The listing builds one solid part. Answer for the finished solid, in the listing's coordinates (mm). A direction names the side the tool comes from. Coordinates: 2 decimals unless noted, no trailing zeros. Write each loop counter-clockwise with the first axis right and the second up, starting at its lowest first coordinate (ties: lowest second). Pieces come first, ordered by that corner, then holes.
(1) For a pull along Y with two mould halves and no side action, classify faces 4 (the cylindrical face through (15.376, 0.066, 6.365)), 5 (the cylindrical face through (12.5, 2.24, -0.05)), 6 (the cylindrical face through (-19.974, -0.068, -6.365)), 7 (the cylindrical face through (6.365, 0.066, -15.376)) as +Y half, -Y half, draft (parallel to the pull), parting line (faces both ways), or undercut.
(2) The part is cut by section A-A on z = 0. Determine the outline of the cut face in (x, y), plus the area to 3 significant figures.
(3) The part is cut by section C-C on z = 5.5. Determine the outline of the cut face in (x, y) (3 decimals), plus the area to 3 significant figures.
(4) The part is cut by section D-D on y = -1. Give the number of separate pieces and of enclosed holes in the cut face, plus the area to 3 significant figures.
(5) The part is cut by section B-B on x = 16. Determine the outline of the cut face in (y, z).
(6) Which of the six approach directions +Z, -Z, +X, -X, +Y, -Y give full straight-line access (tool end or side, diameter ignored) to faces 1 (the cylindrical face through (12.5, -2.24, -0.05)), 2 (the cylindrical face through (-12.5, -2.24, 0.05)), 3 (the cylindrical face through (0.05, 2.24, 12.5))?
(7) Straight lines are drawn through the part: line 1 (X direction, y = 0, z = 7.45) (3 decimals); line 2 (X direction, y = 2.75, z = 15.5). For each, find the intervals that lie inside material, in ascending order.
(8) Given P1, Ø10, axis at x = -16, z = -14.5, coming from the -Y side; P2, Ø1.9, axis at x = -17.5, y = -1, coming from the -Z side; P3, Ø2, axis at y = -1.5, z = 12.5, coming from the -X side; P4, Ø1, axis at y = -2, z = -7.5, coming from the -X side, each flat-ended and moving along its own axis, determine where each tip first touches the part or whether it passes through.
from build123d import *

# Parameters (mm, degrees)
SKETCH1_R           = 2.5
BOSS_EXTRUDE1_DEPTH = 3.1
CUT_EXTRUDE1_START  = -30.25
SKETCH2_R           = 1.5
CUT_EXTRUDE1_DEPTH  = 42.7
CIRPATTERN1_COUNT   = 4
FILLET1_R           = 3
CHAMFER1_SIZE       = 1
CHAMFER3_SIZE       = 0.5


with BuildPart() as part:
    # Sketch1 → Boss-Extrude1 (new body, symmetric)
    with BuildSketch(Plane(origin=(0, 0, 0), x_dir=(1, 0, 0), z_dir=(0, 1, 0))):
        Polygon((-8.9, -13.4), (-8.9, -20.35), (-3.9, -20.35), (-3.9, -13.4), (3.9, -13.4), (3.9, -20.35), (8.9, -20.35), (8.9, -13.4), (13.4, -8.9), (20.35, -8.9), (20.35, -3.9), (13.4, -3.9), (13.4, 3.9), (20.35, 3.9), (20.35, 8.9), (13.4, 8.9), (8.9, 13.4), (8.9, 20.35), (3.9, 20.35), (3.9, 13.4), (-3.9, 13.4), (-3.9, 20.35), (-8.9, 20.35), (-8.9, 13.4), (-13.4, 8.9), (-20.35, 8.9), (-20.35, 3.9), (-13.4, 3.9), (-13.4, -3.9), (-20.35, -3.9), (-20.35, -8.9), (-13.4, -8.9), align=None)
        Circle(SKETCH1_R, mode=Mode.SUBTRACT)
    extrude(amount=BOSS_EXTRUDE1_DEPTH, both=True)

    # Sketch2 → Cut-Extrude1 (cut)
    with BuildSketch(Plane.ZY.offset(8.9).offset(CUT_EXTRUDE1_START)):
        with Locations((16.875, 0)):
            Circle(SKETCH2_R)
        with BuildLine():
            Line((16.875, 3.1), (20.35, 3.1))
            Line((20.35, 3.1), (20.35, -3.1))
            Line((20.35, -3.1), (16.875, -3.1))
            ThreePointArc((16.875, -3.1), (19.975, 0), (16.875, 3.1))
        make_face()
    cut_extrude1 = extrude(amount=CUT_EXTRUDE1_DEPTH, mode=Mode.SUBTRACT)

    # CirPattern1: Cut-Extrude1 ×4 about axis
    cirpattern1_axis = Axis((0, 3.1, 0), (0, 1, 0))
    for i in range(1, CIRPATTERN1_COUNT):
        add(cut_extrude1.rotate(cirpattern1_axis, i * 360 / CIRPATTERN1_COUNT), mode=Mode.SUBTRACT)

    # Fillet1
    fillet1_edges = [part.edges().sort_by_distance(p)[0] for p in [
        (-13.4, 3.1, 0),
        (0, 3.1, 13.4),
        (-13.4, -3.1, 0),
        (0, -3.1, -13.4),
        (13.4, -3.1, 0),
        (0, -3.1, 13.4),
        (13.4, 3.1, 0),
        (0, 3.1, -13.4),
    ]]
    fillet(fillet1_edges, radius=FILLET1_R)

    # Chamfer1
    chamfer1_edges = [part.edges().sort_by_distance(p)[0] for p in [
        (-11.15, 3.1, -11.15),
        (-11.15, -3.1, -11.15),
        (11.15, -3.1, -11.15),
        (11.15, 3.1, 11.15),
        (11.15, -3.1, 11.15),
        (-11.15, -3.1, 11.15),
        (-11.15, 3.1, 11.15),
        (11.15, 3.1, -11.15),
    ]]
    chamfer(chamfer1_edges, length=CHAMFER1_SIZE)

    # Chamfer3
    chamfer3_edges = [part.edges().sort_by_distance(p)[0] for p in [
        (-2.5, -3.1, 0),
        (-2.5, 3.1, 0),
    ]]
    chamfer(chamfer3_edges, length=CHAMFER3_SIZE)


solid = part.part
Model answer:
1. face 4: undercut
1. face 5: +Y half
1. face 6: parting line
1. face 7: undercut
2. outline: (-13.4, -0.1) arc R3 ccw to (-10.4, -3.1) - (-3, -3.1) - (-2.5, -2.6) - (-2.5, 2.6) - (-3, 3.1) - (-10.4, 3.1) arc R3 ccw to (-13.4, 0.1) - close; (2.5, -2.6) - (3, -3.1) - (10.4, -3.1) arc R3 ccw to (13.4, -0.1) - (13.4, 0.1) arc R3 ccw to (10.4, 3.1) - (3, 3.1) - (2.5, 2.6) - close
2. area: 127 mm2
3. outline: (-16.875, -3.1) - (16.875, -3.1) arc R3.1 ccw to (16.875, 3.1) - (-16.875, 3.1) arc R3.1 ccw to start; hole circle Ø3 at (-16.875, 0); hole circle Ø3 at (16.875, 0)
3. area: 225 mm2
4. separate pieces: 9
4. enclosed holes: 1
4. area: 821 mm2
5. outline: (-3.1, -8.9) - (-1.22, -8.9) - (-1.22, -3.9) - (-3.1, -3.9) - close; (-3.1, 3.9) - (-1.22, 3.9) - (-1.22, 8.9) - (-3.1, 8.9) - close; (1.22, -8.9) - (3.1, -8.9) - (3.1, -3.9) - (1.22, -3.9) - close; (1.22, 3.9) - (3.1, 3.9) - (3.1, 8.9) - (1.22, 8.9) - close
6. face 1: +X, -Y
6. face 2: -X, -Y
6. face 3: +Z, +Y
7. line 1: x = -19.975 to -18.375, -15.375 to 15.375, 18.375 to 19.975
7. line 2: x = -8.9 to -3.9, 3.9 to 8.9
8. P1: passes through
8. P2: stops at z = -8.9
8. P3: stops at x = -10.8
8. P4: stops at x = -19.59
